CAD build for the part. Positions are in the model's coordinates, mm. A direction names the side the tool comes from. Round coordinates to 2 decimals unless told otherwise and drop trailing zeros. Order: outer loops, then holes, each group sorted by start corner. A loop starts at its lowest first (then second) coordinate and runs counter-clockwise, first axis right, second up. Notation, with made-up numbers: (-3.75, 70) - (8.25, 70) arc R26 cw to (8.25, 98) - close; hole circle Ø7 at (11.5, 62). An arc over 180 degrees is marked (long way). Write item = value, one per line.
from build123d import *

# Parameters (mm, degrees)
F1_DEPTH = 40


with BuildPart() as f1:
    # F0 (on Front) → F1 (new body)
    with BuildSketch(Plane.XZ):
        Polygon((0, 30), (16, 30), (16, 15), (19, 15), (19, 30), (19, 33), (0, 33), (-3, 33), (-3, 30), (-3, -15), (-40, -15), (-40, 0), (-43, 0), (-43, -18), (-40, -18), (0, -18), (0, -15), align=None)
    extrude(amount=F1_DEPTH)


solid = f1.part
(1) Band-saw the part on B-B on y = -20.5. List the corners of the cut face in (x, z).
Solved:
outline = (-43, -18) - (0, -18) - (0, 30) - (16, 30) - (16, 15) - (19, 15) - (19, 33) - (-3, 33) - (-3, -15) - (-40, -15) - (-40, 0) - (-43, 0) - close
(2) Band-saw the part on C-C on z = 9. List the corners of the cut face in (x, y).
Solved:
outline = (-3, -40) - (0, -40) - (0, 0) - (-3, 0) - close
(3) Band-saw the part on D-D on x = -13.5. List the corners of the cut face in (y, z), plus the area to 3 significant figures.
Solved:
outline = (-40, -18) - (0, -18) - (0, -15) - (-40, -15) - close
area = 120 mm²
(4) Drop flat-ended pins along their axis: pin 1 (0.9 mm diameter, centred on x = -41, y = -14, fed in from +Z); pin 2 (2.5 mm diameter, centred on x = 17, y = -13, fed in from -Z); pin 3 (7.5 mm diameter, centred on y = -14, z = -9, fed in from +X). Give the stop position or say it passes through.
Solved:
pin_1 = 0
pin_2 = 15
pin_3 = 0
(5) Band-saw the part on A-A on z = -4. List the corners of the cut face in (x, y).
Solved:
outline = (-43, -40) - (-40, -40) - (-40, 0) - (-43, 0) - close; (-3, -40) - (0, -40) - (0, 0) - (-3, 0) - close
(6) Pull direction X, two halves, no side cores. Call faces 1 (the flat face through (-41, -20, 0)), 2 (the flat face through (-21, -20, -15)), 3 (the flat face through (-43, -20, -9)): released by +X, released by -X, zero draft, split by the parting line, or undercut.
Solved:
face_1 = zero draft
face_2 = undercut
face_3 = released by -X
(7) Probe line 1 along X through (y, z) = (-13, 23); line 2 along X through (y, z) = (-30, -5); line 3 along Z through (x, y) = (15, -5.5). List the from-to ranges inside material, lowest first.
Solved:
line_1 = -3 to 0, 16 to 19
line_2 = -43 to -40, -3 to 0
line_3 = 30 to 33
(8) Tool access for faces 4 (the flat face through (8, -20, 30)), 5 (the flat face through (-3, -20, 9)), 6 (the flat face through (17, -20, 15)): list every direction of +Z, -Z, +X, -X, +Y, -Y with a clear straight run to the whole face (end or side of a thin tool).
Solved:
face_4 = -Z, +Y, -Y
face_5 = +Z, +Y, -Y
face_6 = -Z, +X, +Y, -Y
